```python
from build123d import *

# Parameters (mm, degrees)
F0_R     = 1.4
F1_DEPTH = 6
F2_R     = 3
F3_R     = 1.35
F4_DEPTH = 75.501


with BuildPart() as f1:
    # F0 (on Front) → F1 (new body)
    with BuildSketch(Plane.XZ):
        with BuildLine():
            Line((-31, 4), (-31, -3))
            Line((-31, -3), (31, -3))
            Line((31, -3), (31, 4))
            ThreePointArc((31, 4), (30.292893, 5.707107), (32, 5))
            Line((32, 5), (42, 5))
            ThreePointArc((42, 5), (43.418637, 5.356618), (44.5, 6.341688))
            Line((44.5, 6.341688), (44.5, 9.658312))
            ThreePointArc((44.5, 9.658312), (43.418637, 10.643382), (42, 11))
            Line((42, 11), (26, 11))
            Line((26, 11), (26, 5))
            Line((26, 5), (26, 3))
            Line((26, 3), (-26, 3))
            Line((-26, 3), (-26, 5))
            Line((-26, 5), (-26, 11))
            Line((-26, 11), (-42, 11))
            ThreePointArc((-42, 11), (-43.418637, 10.643382), (-44.5, 9.658312))
            Line((-44.5, 9.658312), (-44.5, 6.341688))
            ThreePointArc((-44.5, 6.341688), (-43.418637, 5.356618), (-42, 5))
            Line((-42, 5), (-32, 5))
            ThreePointArc((-32, 5), (-30.292893, 5.707107), (-31, 4))
        make_face()
        with Locations((-42, 8)):
            Circle(F0_R, mode=Mode.SUBTRACT)
        with Locations((42, 8)):
            Circle(F0_R, mode=Mode.SUBTRACT)
    extrude(amount=F1_DEPTH)

    # F2
    f2_edges = [f1.edges().sort_by_distance(p)[0] for p in [
        (-26, -3, 11),
        (26, -3, 11),
        (-26, -3, 3),
        (26, -3, 3),
    ]]
    fillet(f2_edges, radius=F2_R)

    # F3 (on face) → F4 (cut, through all)
    with BuildSketch(Plane.YZ.offset(31)):
        with Locations((-3, 0)):
            Circle(F3_R)
    extrude(amount=-F4_DEPTH, mode=Mode.SUBTRACT)


solid = f1.part
```
Read the model definition and answer for the solid it produces. Units are mm, in the model's axes. A direction names the side the tool comes from. Give positions to 0.01 mm unless a question says otherwise; leave off trailing zeros. Write each loop counter-clockwise with the first axis right and the second up, starting at its lowest first coordinate (ties: lowest second). Pieces come first, ordered by that corner, then holes. Notation, with made-up numbers: M 1.25,64 L 24.25,64 A11 ccw 24.25,75 Z; hole C -9.5,5.5 d9. An arc over 180 degrees is marked long. Put each result on its own line as item: value. Start each with the question number.
1. The part is cut by section C-C, the plane x = 36.5. Give the vertices of the cut face in (y, z), and give its area (3 significant figures).
2. Consider line 1 along X through (y, z) = (-5.65, 8.75); line 2 along Z through (x, y) = (-7, -3); line 3 along Z through (x, y) = (42, -1.85). Determine where each line is inside the solid, lowest interval first.
3. The part is cut by section B-B, the plane x = -4.5. Give the vertices of the cut face in (y, z).
4. For a pull along Z with two mould halves and no side action, classify faces 4 (the cylindrical face through (0.434, -1.712, 0.406)), 5 (the cylindrical face through (-26.9, -3.04, 10.14)), 6 (the flat face through (44.5, -3, 8)), 7 (the cylindrical face through (-40.71, -2.96, 7.46)) as released by +Z, released by -Z, zero draft, split by the parting line, or undercut.
5. The part is cut by section A-A, the plane y = -3. Give the vertices of the cut face in (x, z), and give its area (3 significant figures).
6. Each of these flat-tipped pins is pushed along its axis until it touches: pin 1 Ø2 at (y, z) = (-2, 4.5) entering from -X; pin 2 Ø3 at (y, z) = (-3.5, 2) entering from +X; pin 3 Ø1.8 at (x, z) = (-31, 5) entering from +Y. Where does it stop, or does it pass through?
7. Which of the six approach directions +Z, -Z, +X, -X, +Y, -Y give full straight-line access (tool end or side, diameter ignored) to faces 1 (the cylindrical face through (-43.44, -2.96, 5.37)), 2 (the flat face through (31, -3, 2)), 3 (the cylindrical face through (26.9, -3.04, 10.14))?
Final values:
1. outline: M -6,5 L 0,5 L 0,11 L -6,11 Z
1. area: 36.0 mm²
2. line 1: x = -44.5 to -43.18, -40.82 to -26.1, 26.1 to 40.82, 43.18 to 44.5
2. line 2: z = -3 to -1.35, 1.35 to 3
2. line 3: z = 5 to 6.6, 9.4 to 11
3. outline: M -6,-3 L 0,-3 L 0,3 L -6,3 Z; hole C -3,0 d2.7
4. face 4: undercut
4. face 5: released by +Z
4. face 6: zero draft
4. face 7: undercut
5. outline: M -44.5,6.34 A3 ccw -42,5 L -32,5 A1 cw long -31,4 L -31,1.35 L 31,1.35 L 31,4 A1 cw long 32,5 L 42,5 A3 ccw 44.5,6.34 L 44.5,9.66 A3 ccw 42,11 L 29,11 A3 ccw 26,8 L 26,6 A3 cw 23,3 L -23,3 A3 cw -26,6 L -26,8 A3 ccw -29,11 L -42,11 A3 ccw -44.5,9.66 Z; M -31,-3 L 31,-3 L 31,-1.35 L -31,-1.35 Z; hole C -42,8 d2.8; hole C 42,8 d2.8
5. area: 426 mm²
6. pin 1: stops at x = -43.66
6. pin 2: stops at x = 31
6. pin 3: passes through
7. face 1: -Z, -X, +Y, -Y
7. face 2: -Z, +X, +Y, -Y
7. face 3: +Z, +Y, -Y
